Read the model definition and answer for the solid it produces. Units are mm, in the model's axes. Face numbers are marked on the shaded views. Give positions to 0.01 mm unless a question says otherwise; leave off trailing zeros. Loops run counter-clockwise (first coordinate to the right, second up) from the corner with the lowest first, then second, coordinate; pieces in that order, holes last.
(1) Straight lines are drawn through the part: probe 1 along Y at (x, z) = (0, 5); probe 2 along Z at (x, y) = (-4, 16); probe 3 along Y at (x, z) = (0, 7.75). For each, find the intervals that lie inside material, in ascending order.
(2) Determine the mould class of the marked faces 1, 2 and 3 for opening direction Y: pulls with the +Y half, pulls with the -Y half, needs draft (parallel to the pull), parting line crosses it, or undercut.
(3) Each of these flat-tipped pins is pushed along its axis until it touches: P1, Ø10, axis at x = 4, y = -3.5, coming from the -Z side; P2, Ø1.5, axis at y = -14.5, z = 2, coming from the +X side; P3, Ø1, axis at x = -24, y = 4.5, coming from the +Z side; P4, Ø5, axis at x = 16, z = 7, coming from the -Y side. Where does it stop, or does it pass through?
(4) Find section A-A, the plane y = 0. Write down the section's boundary in (x, z).
```python
from build123d import *

# Parameters (mm, degrees)
F0_R     = 32.5
F1_DEPTH = 10
F2_R     = 2.5
F3_T     = -1.5
F4_R     = 32.5
F4_R_2   = 31.75
F5_DEPTH = 2.5


# Not quite as in the source:
# - a feature names something its author has since deleted; it is built from what else it names


with BuildPart() as f1:
    # F0 (on Top) → F1 (new body)
    with BuildSketch(Plane.XY):
        Circle(F0_R)
    extrude(amount=F1_DEPTH)

    # F2
    f2_edges = [f1.edges().sort_by_distance(p)[0] for p in [
        (-32.5, 0, 0),
    ]]
    fillet(f2_edges, radius=F2_R)

    # F3
    f3_openings = [f1.faces().sort_by_distance(p)[0] for p in [
        (0, 0, 10),
    ]]
    offset(amount=F3_T, openings=f3_openings)

    # F4 (on face) → F5 (cut)
    with BuildSketch(Plane.XY.offset(10)):
        Circle(F4_R)
        Circle(F4_R_2, mode=Mode.SUBTRACT)
    extrude(amount=-F5_DEPTH, mode=Mode.SUBTRACT)


solid = f1.part
```
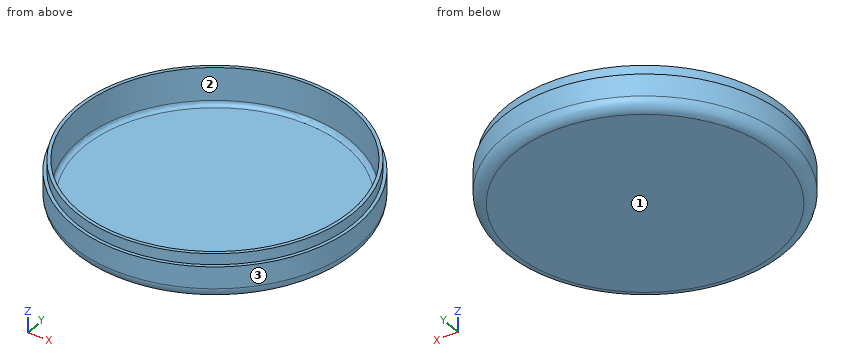
Entries:
1. probe 1: y = -32.5 to -31, 31 to 32.5
1. probe 2: z = 0 to 1.5
1. probe 3: y = -31.75 to -31, 31 to 31.75
2. face 1: needs draft
2. face 2: undercut
2. face 3: parting line crosses it
3. P1: stops at z = 0
3. P2: stops at x = 29.42
3. P3: stops at z = 1.5
3. P4: stops at y = -29.56
4. outline: (-32.5, 2.5) arc R2.5 ccw to (-30, 0) - (30, 0) arc R2.5 ccw to (32.5, 2.5) - (32.5, 7.5) - (31.75, 7.5) - (31.75, 10) - (31, 10) - (31, 2.5) arc R1 cw to (30, 1.5) - (-30, 1.5) arc R1 cw to (-31, 2.5) - (-31, 10) - (-31.75, 10) - (-31.75, 7.5) - (-32.5, 7.5) - close
